Work out the finished part from the listing and answer in its coordinate system (mm). A direction names the side the tool comes from. Coordinates: 2 decimals unless noted, no trailing zeros. Order: outer loops, then holes, each group sorted by start corner. A loop starts at its lowest first (then second) coordinate and runs counter-clockwise, first axis right, second up. Notation, with made-up numbers: (48, 50.5) -> (85, 50.5) arc R31 ccw to (85, 80.5) -> close; hole circle Ø3 at (57, 20). An arc over 180 degrees is marked (long way). Use one line per item in the form item = value.
from build123d import *

# Parameters (mm, degrees)
F0_W     = 125
F0_H     = 100
F1_DEPTH = 6
F2_SIZE  = 10
F3_R     = 1
F4_R     = 6.8
F5_DEPTH = 3


with BuildPart() as f1:
    # F0 (on Top) → F1 (new body)
    with BuildSketch(Plane.XY):
        Rectangle(F0_W, F0_H)
    extrude(amount=F1_DEPTH)

    # F2
    f2_edges = [f1.edges().sort_by_distance(p)[0] for p in [
        (-62.5, 50, 3),
    ]]
    chamfer(f2_edges, length=F2_SIZE)

    # F3
    f3_edges = [f1.edges().sort_by_distance(p)[0] for p in [
        (-62.5, -5, 6),
        (0, -50, 6),
        (62.5, 0, 6),
        (5, 50, 6),
        (-57.5, 45, 6),
    ]]
    fillet(f3_edges, radius=F3_R)

    # F4 (on face) → F5 (cut)
    with BuildSketch(Plane.XY.offset(6)):
        with Locations((46.5, 37)):
            Circle(F4_R)
        with Locations((46.5, 19)):
            Circle(F4_R)
        with Locations((23.5, 37)):
            Circle(F4_R)
        with Locations((23.5, 19)):
            Circle(F4_R)
        with Locations((0.5, 37)):
            Circle(F4_R)
        with Locations((0.5, 19)):
            Circle(F4_R)
        with Locations((46.5, 1)):
            Circle(F4_R)
        with Locations((46.5, -17)):
            Circle(F4_R)
        with Locations((23.5, 1)):
            Circle(F4_R)
        with Locations((23.5, -17)):
            Circle(F4_R)
        with Locations((0.5, 1)):
            Circle(F4_R)
        with Locations((0.5, -17)):
            Circle(F4_R)
        with Locations((-22.5, 37)):
            Circle(F4_R)
        with Locations((-22.5, 19)):
            Circle(F4_R)
        with Locations((-22.5, 1)):
            Circle(F4_R)
        with Locations((-22.5, -17)):
            Circle(F4_R)
        with Locations((-45.5, 37)):
            Circle(F4_R)
        with Locations((-45.5, 19)):
            Circle(F4_R)
        with Locations((-45.5, 1)):
            Circle(F4_R)
        with Locations((-45.5, -17)):
            Circle(F4_R)
        with Locations((46.5, -35)):
            Circle(F4_R)
        with Locations((23.5, -35)):
            Circle(F4_R)
        with Locations((0.5, -35)):
            Circle(F4_R)
        with Locations((-22.5, -35)):
            Circle(F4_R)
        with Locations((-45.5, -35)):
            Circle(F4_R)
    extrude(amount=-F5_DEPTH, mode=Mode.SUBTRACT)


solid = f1.part
(1) Section A-A on y = 19 is taken. Write down the section's boundary in (x, z).
Data:
outline = (-62.5, 0) -> (62.5, 0) -> (62.5, 5) arc R1 ccw to (61.5, 6) -> (53.3, 6) -> (53.3, 3) -> (39.7, 3) -> (39.7, 6) -> (30.3, 6) -> (30.3, 3) -> (16.7, 3) -> (16.7, 6) -> (7.3, 6) -> (7.3, 3) -> (-6.3, 3) -> (-6.3, 6) -> (-15.7, 6) -> (-15.7, 3) -> (-29.3, 3) -> (-29.3, 6) -> (-38.7, 6) -> (-38.7, 3) -> (-52.3, 3) -> (-52.3, 6) -> (-61.5, 6) arc R1 ccw to (-62.5, 5) -> close
(2) Section B-B on x = 46.5 is taken. Write down the section's boundary in (y, z).
Data:
outline = (-50, 0) -> (50, 0) -> (50, 5) arc R1 ccw to (49, 6) -> (43.8, 6) -> (43.8, 3) -> (30.2, 3) -> (30.2, 6) -> (25.8, 6) -> (25.8, 3) -> (12.2, 3) -> (12.2, 6) -> (7.8, 6) -> (7.8, 3) -> (-5.8, 3) -> (-5.8, 6) -> (-10.2, 6) -> (-10.2, 3) -> (-23.8, 3) -> (-23.8, 6) -> (-28.2, 6) -> (-28.2, 3) -> (-41.8, 3) -> (-41.8, 6) -> (-49, 6) arc R1 ccw to (-50, 5) -> close
(3) Which of the six approach directions +Z, -Z, +X, -X, +Y, -Y give full straight-line access (tool end or side, diameter ignored) to faces 5 (the flat face through (62.5, -1, 2)), 6 (the cylindrical face through (-39.219, -19.604, 4.521))?
Data:
face_5 = +Z, -Z, +X, +Y, -Y
face_6 = +Z
(4) Straight lines are drawn through the part: line 1 along Y through (x, z) = (46.5, 4.95); line 2 along Y through (x, z) = (-49, 3.8); line 3 along X through (y, z) = (31, 3.95). For each, find the intervals that lie inside material, in ascending order.
Data:
line_1 = -50 to -41.8, -28.2 to -23.8, -10.2 to -5.8, 7.8 to 12.2, 25.8 to 30.2, 43.8 to 50
line_2 = -50 to -40.83, -29.17 to -22.83, -11.17 to -4.83, 6.83 to 13.17, 24.83 to 31.17, 42.83 to 50
line_3 = -62.5 to -48.7, -42.3 to -25.7, -19.3 to -2.7, 3.7 to 20.3, 26.7 to 43.3, 49.7 to 62.5
(5) The mould has two halves that part along X. Classify faces 1 (the cylindrical face through (52.781, 16.396, 4.521)), 2 (the flat face through (4, 50, 2)), 3 (the flat face through (-46, 1, 3)), 4 (the cylindrical face through (-57.228, 44.868, 5.699)): released by +X, released by -X, zero draft, split by the parting line, or undercut.
Data:
face_1 = undercut
face_2 = zero draft
face_3 = undercut
face_4 = released by -X
